Read the model definition and answer for the solid it produces. Units are mm, in the model's axes. Round coordinates to 2 decimals unless told otherwise and drop trailing zeros. Order: outer loops, then holes, each group sorted by start corner. A loop starts at its lowest first (then second) coordinate and runs counter-clockwise, first axis right, second up. Notation, with made-up numbers: (-2, 44.5) - (23, 44.5) arc R18 ccw to (23, 62.5) - close; hole circle Ø11 at (-17.5, 86). An arc over 180 degrees is marked (long way). Answer as a JSON object with one key per item and string values. Group by question number.
Q1. Given pin 1 Ø8 at (y, z) = (-8.5, 341.5) entering from -X; pin 2 Ø9.5 at (y, z) = (-14, 326.5) entering from +X; pin 3 Ø10 at (y, z) = (-12.5, 79.5) entering from +X, each flat-ended and moving along its own axis, determine where each tip first touches the part or whether it passes through.
Q2. Consider line 1 (Z direction, x = -110.5, y = -11.5) (3 decimals); line 2 (X direction, y = -12, z = -112.5); line 3 (X direction, y = -1.5, z = -60). Determine where each line is inside the solid, lowest interval first.
Q3. A cutting plane is placed at A-A on z = -14. Determine the outline of the cut face in (x, y), and give its area (3 significant figures).
```python
from build123d import *

# Parameters (mm, degrees)
F1_DEPTH = 19.05
F2_R     = 38.1
F3_R     = 5.08
F4_R     = 5.08
F5_SIZE  = 1.5875


with BuildPart() as f1:
    # F0 (on Front) → F1 (new body)
    with BuildSketch(Plane.XZ):
        Polygon((50.8, -288.925), (50.8, 288.925), (171.45, 288.925), (171.45, 365.125), (9.525, 365.125), (9.525, 288.925), (-9.525, 288.925), (-9.525, 365.125), (-171.45, 365.125), (-171.45, 288.925), (-50.8, 288.925), (-50.8, -288.925), (-209.55, -288.925), (-209.55, -365.125), (-95.25, -365.125), (-95.25, -358.775), (-9.525, -358.775), (-9.525, -282.575), (9.525, -282.575), (9.525, -358.775), (95.25, -358.775), (95.25, -365.125), (209.55, -365.125), (209.55, -288.925), align=None)
    extrude(amount=F1_DEPTH)

    # F2
    f2_edges = [f1.edges().sort_by_distance(p)[0] for p in [
        (50.8, -9.525, 288.925),
        (-50.8, -9.525, 288.925),
        (171.45, -9.525, 288.925),
        (-171.45, -9.525, 288.925),
        (-209.55, -9.525, -288.925),
        (50.8, -9.525, -288.925),
        (209.55, -9.525, -288.925),
        (-50.8, -9.525, -288.925),
    ]]
    fillet(f2_edges, radius=F2_R)

    # F3
    f3_edges = [f1.edges().sort_by_distance(p)[0] for p in [
        (9.525, -9.525, 288.925),
        (-9.525, -9.525, 288.925),
    ]]
    fillet(f3_edges, radius=F3_R)

    # F4
    f4_edges = [f1.edges().sort_by_distance(p)[0] for p in [
        (9.525, -9.525, -282.575),
        (-9.525, -9.525, -282.575),
    ]]
    fillet(f4_edges, radius=F4_R)

    # F5
    f5_edges = [f1.edges().sort_by_distance(p)[0] for p in [
        (-50.8, -19.05, 0),
        (-50.8, 0, 0),
        (50.8, -19.05, 0),
        (50.8, 0, 0),
    ]]
    chamfer(f5_edges, length=F5_SIZE)


solid = f1.part
```
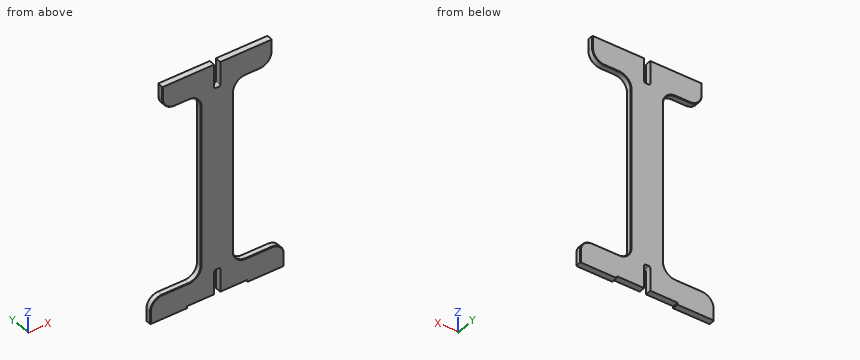
Result set:
{
 "1": {"pin 1": "stops at x = -171.45", "pin 2": "stops at x = 171.45", "pin 3": "stops at x = 50.8"},
 "2": {"line 1": "z = -365.125 to -288.925, 288.925 to 365.125", "line 2": "x = -50.8 to 50.8", "line 3": "x = -50.71 to 50.71"},
 "3": {"outline": "(-50.8, -17.46) - (-49.21, -19.05) - (49.21, -19.05) - (50.8, -17.46) - (50.8, -1.59) - (49.21, 0) - (-49.21, 0) - (-50.8, -1.59) - close", "area": "1,930 mm²"}
}
